Autodesk Inventor part; units mm, degrees
ref_plane "YZ Plane" through (0, 0, 0) normal (1, 0, 0) x (0, 1, 0)
ref_plane "XZ Plane" through (0, 0, 0) normal (0, 1, 0) x (-1, 0, 0)
ref_plane "XY Plane" through (0, 0, 0) normal (0, 0, 1) x (1, 0, 0)
sketch "Sketch1" plane through (0, 0, 0) normal (0, 1, 0) x (-1, 0, 0)
  circle A0 centre (0, 0) radius 75
  circle A1 centre (0, 65.8304) radius 2.8396
  circle A2 centre (-46.5491, 46.5491) radius 2.8396
  circle A3 centre (-65.8304, 0) radius 2.8396
  circle A4 centre (-46.5491, -46.5491) radius 2.8396
  circle A5 centre (0, -65.8304) radius 2.8396
  circle A6 centre (46.5491, -46.5491) radius 2.8396
  circle A7 centre (65.8304, 0) radius 2.8396
  circle A8 centre (46.5491, 46.5491) radius 2.8396
  line L0 (-21.1442, 51.6217) -> (21.1442, 51.6217)
  line L1 (21.1442, 51.6217) -> (21.1442, 48.6217)
  line L2 (21.1442, 48.6217) -> (-21.1442, 48.6217)
  line L3 (-21.1442, 48.6217) -> (-21.1442, 51.6217)
  line L4 (-21.1442, 51.6217) -> (21.1442, 48.6217) construction
  line L5 (21.1442, 51.6217) -> (-21.1442, 48.6217) construction
  line L6 (-21.1442, 46.6217) -> (21.1442, 46.6217)
  line L7 (21.1442, 46.6217) -> (21.1442, 43.6217)
  line L8 (21.1442, 43.6217) -> (-21.1442, 43.6217)
  line L9 (-21.1442, 43.6217) -> (-21.1442, 46.6217)
  line L10 (-21.1442, 46.6217) -> (21.1442, 43.6217) construction
  line L11 (21.1442, 46.6217) -> (-21.1442, 43.6217) construction
  line L12 (-21.1442, 41.6217) -> (21.1442, 41.6217)
  line L13 (21.1442, 41.6217) -> (21.1442, 38.6217)
  line L14 (21.1442, 38.6217) -> (-21.1442, 38.6217)
  line L15 (-21.1442, 38.6217) -> (-21.1442, 41.6217)
  line L16 (-21.1442, 41.6217) -> (21.1442, 38.6217) construction
  line L17 (21.1442, 41.6217) -> (-21.1442, 38.6217) construction
  line L18 (-21.1442, 36.6217) -> (21.1442, 36.6217)
  line L19 (21.1442, 33.6217) -> (-21.1442, 33.6217)
  line L20 (-21.1442, 33.6217) -> (-21.1442, 36.6217)
  line L21 (-21.1442, 36.6217) -> (21.1442, 33.6217) construction
  line L22 (21.1442, 36.6217) -> (-21.1442, 33.6217) construction
  line L23 (-21.1442, 31.6217) -> (21.1442, 31.6217)
  line L24 (21.1442, 28.6217) -> (-21.1442, 28.6217)
  line L25 (-21.1442, 28.6217) -> (-21.1442, 31.6217)
  line L26 (-21.1442, 31.6217) -> (21.1442, 28.6217) construction
  line L27 (21.1442, 31.6217) -> (-21.1442, 28.6217) construction
  line L28 (21.1442, 36.6217) -> (21.1442, 33.6217)
  line L29 (21.1442, 31.6217) -> (21.1442, 28.6217)
  point P0 (0, 50.1217)
  point P1 (0, 45.1217)
  point P2 (0, 40.1217)
  point P3 (0, 35.1217)
  point P4 (0, 30.1217)
  dimension "d0" = 150
  dimension "d3" = 360
  dimension "d5" = 3
  dimension "d6" = 3
  dimension "d7" = 3
  dimension "d8" = 2
  dimension "d9" = 2
  dimension "d12" = 3
  dimension "d15" = 3
  dimension "d16" = 2
  dimension "d17" = 2
extrude "Extrusion1" add sketch "Sketch1" along normal blind 4
sketch "Sketch2" plane through (0, 4, 0) normal (0, 1, 0) x (1, 0, 0)
  point P0 (0, 0)
properties part number "Baseplate"
For this review, take the finished solid that the model builds, in its own axes (mm). Round coordinates to 2 decimals unless told otherwise and drop trailing zeros. Loops run counter-clockwise (first coordinate to the right, second up) from the corner with the lowest first, then second, coordinate; pieces in that order, holes last. Notation, with made-up numbers: (69.5, 72) - (120.5, 72) arc R11 cw to (120.5, 82) - close; hole circle Ø1 at (-34.5, 20). An arc over 180 degrees is marked (long way). One line per question, with ' | ' between items.
Q1. Take a section at C-C (x = -65.5). Give the boundary of the cut face in (y, z), and give its area (3 significant figures).
Taken from the geometry:
outline: (0, -36.53) - (4, -36.53) - (4, -2.82) - (0, -2.82) - close; (0, 2.82) - (4, 2.82) - (4, 36.53) - (0, 36.53) - close | area: 270 mm²
Q2. Take a section at B-B (z = 0). Give the boundary of the cut face in (x, y), and give its area (3 significant figures).
Taken from the geometry:
outline: (-75, 0) - (-68.67, 0) - (-68.67, 4) - (-75, 4) - close; (-62.99, 0) - (62.99, 0) - (62.99, 4) - (-62.99, 4) - close; (68.67, 0) - (75, 0) - (75, 4) - (68.67, 4) - close | area: 555 mm²
Q3. For line 1 along X through (y, z) = (3.15, 48.5); line 2 along Z through (x, y) = (-11.5, 3.5); line 3 along Z through (x, y) = (16.5, 2.6), list the stretches that pass through material, from the lowest coordinate up. Write a range as [from, to].
Taken from the geometry:
line 1: x = [-57.21, -48.61], [-44.49, 44.49], [48.61, 57.21] | line 2: z = [-74.11, 28.62], [31.62, 33.62], [36.62, 38.62], [41.62, 43.62], [46.62, 48.62], [51.62, 74.11] | line 3: z = [-73.16, 28.62], [31.62, 33.62], [36.62, 38.62], [41.62, 43.62], [46.62, 48.62], [51.62, 73.16]
Q4. Take a section at A-A (x = 0). State how many separate pieces and enclosed holes the cut face has, and give its area (3 significant figures).
Taken from the geometry:
separate pieces: 8 | enclosed holes: 0 | area: 495 mm²
Q5. For pin 1 (0.9 mm diameter, centred on y = 2, z = 45.5, fed in from -X); pin 2 (2 mm diameter, centred on x = -6, y = 1.5, fed in from +Z); pin 3 (1 mm diameter, centred on y = 2, z = -19.5, fed in from +X); pin 4 (3.5 mm diameter, centred on x = -46.55, z = -46.55, fed in from -Y), all flat-tipped, find the tip position at first contact; note any pin that passes through.
Taken from the geometry:
pin 1: stops at x = -59.96 | pin 2: stops at z = 74.83 | pin 3: stops at x = 72.55 | pin 4: passes through
Q6. The part is to be moulded in two halves that separate along Z. For faces 1 (the cylindrical face through (9.764, 1.972, -74.362)), 2 (the flat face through (1, 4, 1)), 3 (the flat face through (0, 2, 31.622)), 4 (the flat face through (0, 2, 51.622)), say which applies: released by +Z, released by -Z, zero draft, split by the parting line, or undercut.
Taken from the geometry:
face 1: split by the parting line | face 2: zero draft | face 3: undercut | face 4: undercut
